Verification items for this drawing (mm, ordinates from the low corner). Coordinates: 2 decimals unless noted, no trailing zeros. Order: outer loops, then holes, each group sorted by start corner. A loop starts at its lowest first (then second) coordinate and runs counter-clockwise, first axis right, second up. Notation, with made-up numbers: (56, -37) - (71, -37) arc R25 cw to (71, -11) - close; hole circle Ø9 at (7.25, 47.5). An arc over 180 degrees is marked (long way). Use CSV: the item, a comma, the result in double quotes. Start each with the question number.
1) Depth check by flat-ended pin: P1, Ø1.3, axis at y = 1.5, z = 9, coming from the -X side; P2, Ø1.3, axis at x = 30.5, y = 1, coming from the -Z side. Enter the tip coordinate at first touch or a pass-through.
2) Sectioned sample at C-C, the plane z = 37. Record the cut outline in (x, y), and give its area (3 significant figures).
3) Thickness scan on probe 1 along X at (y, z) = (0.3, 36); probe 2 along Z at (x, y) = (24.5, 0.8) (1 decimal). Record the ranges inside material, lowest first. Write a range as [from, to].
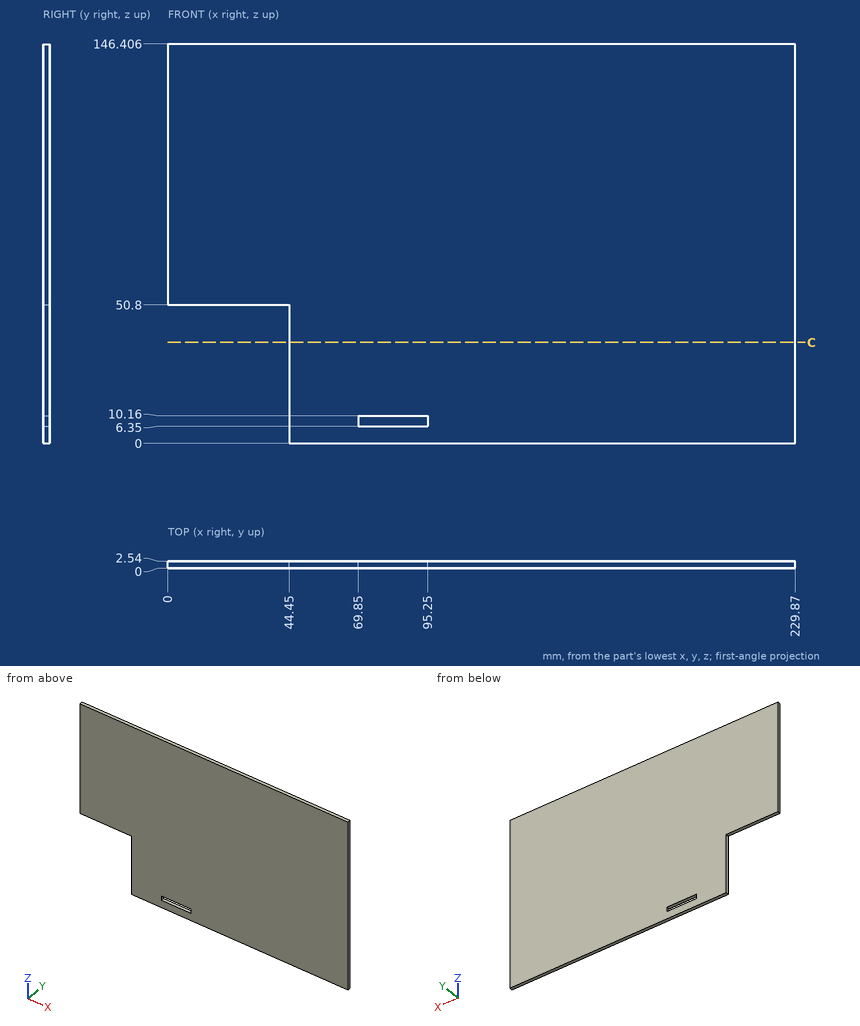
Evaluation:
1,P1,"x = 44.45"
1,P2,"z = 50.8"
2,outline,"(44.45, 0) - (229.87, 0) - (229.87, 2.54) - (44.45, 2.54) - close"
2,area,"471 mm²"
3,probe 1,"[44.45, 229.87]"
3,probe 2,"[50.8, 146.4]"
